Could you check a few things on this model? Use its own coordinates, in mm. A direction names the side the tool comes from. Round coordinates to 2 decimals unless told otherwise and drop trailing zeros. Loops run counter-clockwise (first coordinate to the right, second up) from the corner with the lowest first, then second, coordinate; pieces in that order, holes last. Notation, with made-up numbers: M -13,39.5 L 18,39.5 A13 cw 18,52.5 Z; hole C -24.75,40.25 d2. An arc over 180 degrees is marked long. Answer in a Markdown table with one row per item.
```python
from build123d import *

# Parameters (mm, degrees)
SKETCH1_W                    = 152.4
SKETCH1_H                    = 152.4
BOSS_EXTRUDE1_DEPTH          = 2.6
BOSS_EXTRUDE4_DEPTH          = 152.4
TAP_DRILL_FOR_M8_HELICOIL2_D = 8.25
SKETCH2_R                    = 1.6
CUT_EXTRUDE1_DEPTH           = 3.6


with BuildPart() as part:
    # Sketch1 → Boss-Extrude1 (new body)
    with BuildSketch(Plane.XY):
        with Locations((76.2, 76.2)):
            Rectangle(SKETCH1_W, SKETCH1_H)
    extrude(amount=BOSS_EXTRUDE1_DEPTH)

    # Sketch8 → Boss-Extrude4 (add, through all)
    with BuildSketch(Plane(origin=(0, 152.4, 0), x_dir=(1, 0, 0), z_dir=(0, 1, 0))):
        Polygon((34, -2.6), (46.2, -14.8), (106.2, -14.8), (118.4, -2.6), align=None)
    extrude(amount=-BOSS_EXTRUDE4_DEPTH)

    # Tap Drill for M8 Helicoil2 (through all)
    with Locations(Plane(origin=(0, 152.4, 0), x_dir=(1, 0, 0), z_dir=(0, 1, 0))):
        with Locations((76.2, -8.7)):
            Hole(TAP_DRILL_FOR_M8_HELICOIL2_D / 2)

    # Sketch2 → Cut-Extrude1 (cut, through all)
    with BuildSketch(Plane.XY.offset(2.6)):
        with Locations((5, 128.5)):
            Circle(SKETCH2_R)
        with Locations((29, 146.3)):
            Circle(SKETCH2_R)
        with Locations((5, 146.3)):
            Circle(SKETCH2_R)
        with Locations((29, 128.5)):
            Circle(SKETCH2_R)
        with Locations((123.4, 146.3)):
            Circle(SKETCH2_R)
        with Locations((147.4, 146.3)):
            Circle(SKETCH2_R)
        with Locations((147.4, 128.5)):
            Circle(SKETCH2_R)
        with Locations((123.4, 128.5)):
            Circle(SKETCH2_R)
        with Locations((123.4, 23.9)):
            Circle(SKETCH2_R)
        with Locations((147.4, 23.9)):
            Circle(SKETCH2_R)
        with Locations((147.4, 6.1)):
            Circle(SKETCH2_R)
        with Locations((123.4, 6.1)):
            Circle(SKETCH2_R)
        with Locations((5, 23.9)):
            Circle(SKETCH2_R)
        with Locations((29, 23.9)):
            Circle(SKETCH2_R)
        with Locations((29, 6.1)):
            Circle(SKETCH2_R)
        with Locations((5, 6.1)):
            Circle(SKETCH2_R)
    extrude(amount=-CUT_EXTRUDE1_DEPTH, mode=Mode.SUBTRACT)


solid = part.part
```
1) Will these pins go through, and if not, where does the flat tip stop? P1, Ø10, axis at x = 128, y = 67.5, coming from the +Z side; P2, Ø1.5, axis at y = 16, z = 5.5, coming from the +X side; P3, Ø2, axis at y = 69, z = 7, coming from the -X side.
Computed:
| item | result |
|---|---|
| P1 | stops at z = 2.6 |
| P2 | stops at x = 116.25 |
| P3 | stops at x = 37.4 |
2) If we mould it in two halves opening along Z, with no side actions, what happens to faces 4 (the face through (75, 152.4, 4)), 5 (the face through (73.982, 75.133, 5.222)), 6 (the face through (75, 77, 0))? For each: released by +Z, released by -Z, zero draft, split by the parting line, or undercut.
Computed:
| item | result |
|---|---|
| face 4 | zero draft |
| face 5 | undercut |
| face 6 | released by -Z |
3) Which directions (+Z, -Z, +X, -X, +Y, -Y) give clear straight access to the entire face, cutting with the end or side of a thin tool? Please do faces 1 (the face through (17, 77, 2.6)), 2 (the face through (75, 0, 4)), 3 (the face through (135, 77, 2.6)).
Computed:
| item | result |
|---|---|
| face 1 | +Z, -X, +Y, -Y |
| face 2 | +Z, -Z, +X, -X, -Y |
| face 3 | +Z, +X, +Y, -Y |
4) I want a section at B-B, the plane x = 76.2. Please give me the cut outline in (y, z) (3 decimals), plus the area to 3 significant figures.
Computed:
| item | result |
|---|---|
| outline | M 0,0 L 152.4,0 L 152.4,4.575 L 0,4.575 Z; M 0,12.825 L 152.4,12.825 L 152.4,14.8 L 0,14.8 Z |
| area | 998 mm² |
5) I want a section at C-C, the plane y = 142. Please give me the cut outline in (x, z) (3 decimals).
Computed:
| item | result |
|---|---|
| outline | M 0,0 L 152.4,0 L 152.4,2.6 L 118.4,2.6 L 106.2,14.8 L 46.2,14.8 L 34,2.6 L 0,2.6 Z; hole C 76.2,8.7 d8.25 |
6) I want a section at A-A, the plane z = 6.75. Please give me the cut outline in (x, y).
Computed:
| item | result |
|---|---|
| outline | M 38.15,0 L 72.57,0 L 72.57,152.4 L 38.15,152.4 Z; M 79.83,0 L 114.25,0 L 114.25,152.4 L 79.83,152.4 Z |
7) I need wall thicknesses on line 1 (X direction, y = 128.5, z = 1.7); line 2 (Y direction, x = 5, z = 1.5); line 3 (X direction, y = 24.5, z = 2.5). Which ranges of each line are inside material? Lowest first, please.
Computed:
| item | result |
|---|---|
| line 1 | x = 0 to 3.4, 6.6 to 27.4, 30.6 to 121.8, 125 to 145.8, 149 to 152.4 |
| line 2 | y = 0 to 4.5, 7.7 to 22.3, 25.5 to 126.9, 130.1 to 144.7, 147.9 to 152.4 |
| line 3 | x = 0 to 3.52, 6.48 to 27.52, 30.48 to 121.92, 124.88 to 145.92, 148.88 to 152.4 |
8) I want a section at D-D, the plane x = 39.5. Please give me the cut outline in (y, z), plus the area to 3 significant figures.
Computed:
| item | result |
|---|---|
| outline | M 0,0 L 152.4,0 L 152.4,8.1 L 0,8.1 Z |
| area | 1,230 mm² |
